Geometry check sheet. Reference: drawing and pictorial views, mm from the part's lowest x, y, z. A direction names the side the tool comes from. Coordinates: 2 decimals unless noted, no trailing zeros. Write each loop counter-clockwise with the first axis right and the second up, starting at its lowest first coordinate (ties: lowest second). Pieces come first, ordered by that corner, then holes. Notation, with made-up numbers: (5, 32) -> (35, 32) arc R29 cw to (35, 53) -> close; hole circle Ø7 at (89.5, 81). An arc over 180 degrees is marked (long way). Answer in a Markdown table with one row per item.
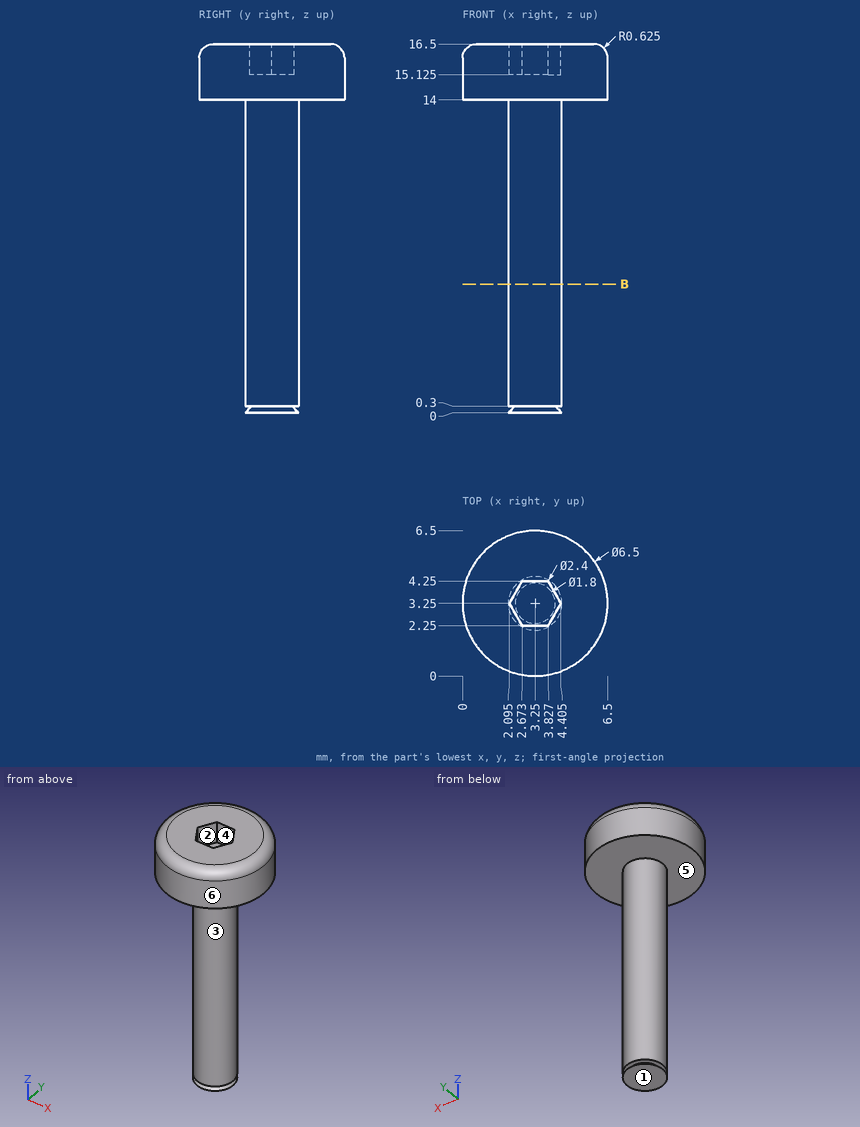
1. Tool access check on the marked faces 5 and 6. Record the directions out of +Z, -Z, +X, -X, +Y, -Y that give a thin tool (end or side, any length) a straight path to the whole face; none if there is none.
Geometry says:
| item | result |
|---|---|
| face 5 | -Z |
| face 6 | +Z, -Z |
2. Section check B-B, the plane z = 5.75. Record the boundary of the cut face in (x, y).
Geometry says:
| item | result |
|---|---|
| outline | circle Ø2.4 at (3.25, 3.25) |
3. Thickness scan on line 1 (Y direction, x = 3.25, z = 10.5); line 2 (Z direction, x = 5, y = 4.75); line 3 (Z direction, x = 3.5, y = 2.5) (1 decimal). Record the ranges inside material, lowest first. Write a range as from..to.
Geometry says:
| item | result |
|---|---|
| line 1 | 2.05..4.45 |
| line 2 | 14..16.5 |
| line 3 | 0..15.1 |
4. Depth check by flat-ended pin: P1, Ø1, axis at y = 3, z = 10, coming from the -X side; P2, Ø2, axis at x = 4, z = 3, coming from the +Y side; P3, Ø1.5, axis at x = 5, y = 1, coming from the -Z side. Enter the tip coordinate at first touch or a pass-through.
Geometry says:
| item | result |
|---|---|
| P1 | x = 2.05 |
| P2 | y = 4.45 |
| P3 | z = 14 |
5. Mould release check, pull along X, two halves, no side actions. Record for the marked faces 1, 2, 3 and 4: released by +X, released by -X, zero draft, split by the parting line, or undercut.
Geometry says:
| item | result |
|---|---|
| face 1 | zero draft |
| face 2 | undercut |
| face 3 | split by the parting line |
| face 4 | undercut |
